```python
from build123d import *

# Parameters (mm, degrees)
FILLET4_R               = 3
CHAMFER1_SIZE2          = 0.393197641
CHAMFER1_SIZE           = 0.4
CUT_EXTRUDE1_DEPTH      = 10.487768718
CUT_EXTRUDE1_DEPTH_BACK = 12.0000001
FILLET5_R               = 0.4
FILLET6_R               = 2


with BuildPart() as part:
    # Sketch1 → Revolve1 (revolve)
    with BuildSketch(Plane.XY):
        Polygon((0, 1.95), (10.718918331, 1.95), (15.775669274, 0.5), (20.487768618, 0.58225), (20.487768618, 2.582554656), (16.03962094, 2.50491195), (11, 3.95), (11, 10), (8, 10), (8, 2.75), (0, 2.75), align=None)
    revolve(axis=Axis((0, 0, 0), (1, 0, 0)))

    # Fillet4
    fillet4_edges = [part.edges().sort_by_distance(p)[0] for p in [
        (15.775669274, -0.5, 0),
        (10.718918331, -1.95, 0),
    ]]
    fillet(fillet4_edges, radius=FILLET4_R)

    # Chamfer1
    chamfer1_edges = [part.edges().sort_by_distance(p)[0] for p in [
        (20.487768618, -2.582554656, 0),
    ]]
    chamfer(chamfer1_edges, length=CHAMFER1_SIZE, length2=CHAMFER1_SIZE2)

    # Sketch2 → Cut-Extrude1 (cut, two sides)
    with BuildSketch(Plane(origin=(11, 0, 0), x_dir=(0, 0, -1), z_dir=(1, 0, 0))) as cut_extrude1_sk:
        with BuildLine():
            Line((-10, 0), (-5, 8.660254038))
            ThreePointArc((-5, 8.660254038), (-8.660254038, 5), (-10, 0))
        make_face()
        with BuildLine():
            Line((-5, 8.660254038), (5, 8.660254038))
            ThreePointArc((5, 8.660254038), (0, 10), (-5, 8.660254038))
        make_face()
        with BuildLine():
            Line((5, 8.660254038), (10, 0))
            ThreePointArc((10, 0), (8.660254038, 5), (5, 8.660254038))
        make_face()
        with BuildLine():
            ThreePointArc((-10, 0), (-8.660254038, -5), (-5, -8.660254038))
            Line((-5, -8.660254038), (-10, 0))
        make_face()
        with BuildLine():
            ThreePointArc((-5, -8.660254038), (0, -10), (5, -8.660254038))
            Line((5, -8.660254038), (-5, -8.660254038))
        make_face()
        with BuildLine():
            ThreePointArc((5, -8.660254038), (8.660254038, -5), (10, 0))
            Line((10, 0), (5, -8.660254038))
        make_face()
    extrude(amount=CUT_EXTRUDE1_DEPTH, mode=Mode.SUBTRACT)
    extrude(cut_extrude1_sk.sketch, amount=-CUT_EXTRUDE1_DEPTH_BACK, mode=Mode.SUBTRACT)

    # Fillet5
    fillet5_edges = [part.edges().sort_by_distance(p)[0] for p in [
        (11, -4.330127019, -7.5),
        (8, -4.330127019, -7.5),
        (8, -8.660254038, 0),
        (8, 4.330127019, -7.5),
        (8, 4.330127019, 7.5),
        (9.5, 8.660254038, 5),
        (11, 4.330127019, 7.5),
        (9.5, 0, 10),
        (9.5, 0, -10),
        (11, 4.330127019, -7.5),
        (9.5, 8.660254038, -5),
        (9.5, -8.660254038, 5),
        (11, -8.660254038, 0),
        (9.5, -8.660254038, -5),
        (11, 8.660254038, 0),
        (8, 8.660254038, 0),
        (11, -4.330127019, 7.5),
        (8, -4.330127019, 7.5),
    ]]
    fillet(fillet5_edges, radius=FILLET5_R)

    # Fillet6
    fillet6_edges = [part.edges().sort_by_distance(p)[0] for p in [
        (11, -3.95, 0),
        (16.03962094, -2.50491195, 0),
    ]]
    fillet(fillet6_edges, radius=FILLET6_R)


solid = part.part
```
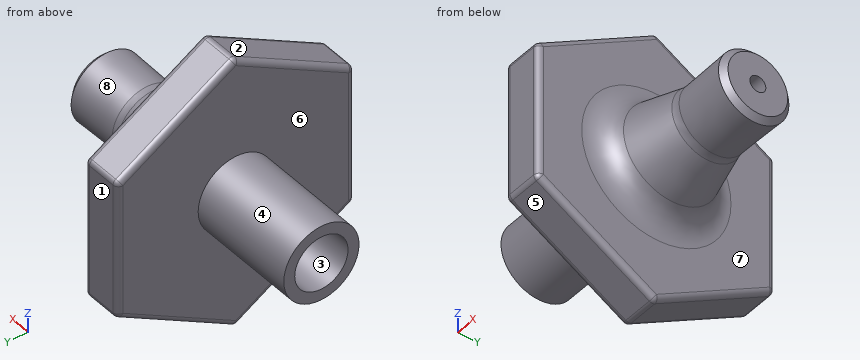
Model file for the job. Use its own axes, mm. Face numbers are marked on the shaded views. A direction names the side the tool comes from. Coordinates: 2 decimals unless noted, no trailing zeros. Write each loop counter-clockwise with the first axis right and the second up, starting at its lowest first coordinate (ties: lowest second). Pieces come first, ordered by that corner, then holes. Notation, with made-up numbers: (-16.5, 21) - (16.5, 21) arc R21 ccw to (16.5, 50) - close; hole circle Ø1 at (61.25, -4). An arc over 180 degrees is marked (long way). One line per question, with ' | ' between items. Start each with the question number.
Q1. Drill centre lines: line 1 (Z direction, x = 6, y = 0); line 2 (X direction, y = 2.25, z = -6.5); line 3 (Z direction, x = 10.25, y = 0.25). Where is each one in solid material? Low to high. Write a range as [from, to].
Q2. Pin check, flat tips, straight feed: pin 1 (3 mm diameter, centred on x = 17.5, z = 2.5, fed in from -Y); pin 2 (5 mm diameter, centred on y = 0, z = 0, fed in from +X); pin 3 (8 mm diameter, centred on y = 7, z = 5, fed in from -X); pin 4 (3 mm diameter, centred on x = 6, z = 7.5, fed in from -Y) (3 decimals). Stop position of each tip, or through.
Q3. Cut at B-B, the plane x = 3.5. List the corners of the cut face in (y, z), then the cut area to 3 significant figures.
Q4. Cut at C-C, the plane x = 19.25. List the corners of the cut face in (y, z).
Q5. Cut at A-A, the plane x = 9. List the corners of the cut face in (y, z), then the cut area to 3 significant figures.
Q6. Pull direction Y, two halves, no side cores. Call the marked faces 1, 2, 3 and 4: pulls with the +Y half, pulls with the -Y half, needs draft (parallel to the pull), parting line crosses it, or undercut.
Q7. 3-axis set-ups, long thin cutter, end or side, ignore diameter. For the marked faces 5, 6, 7 and 8: which of +Z, -Z, +X, -X, +Y, -Y reach the whole face in a straight line?
Answer below:
1) line 1: [-2.75, -1.95], [1.95, 2.75] | line 2: [8, 11] | line 3: [-9.86, -1.93], [1.93, 9.86]
2) pin 1: y = -2.33 | pin 2: x = 20.49 | pin 3: x = 8 | pin 4: through
3) outline: circle Ø5.5 at (0, 0); hole circle Ø3.9 at (0, 0) | area: 11.8 mm^2
4) outline: circle Ø5.12 at (0, 0); hole circle Ø1.12 at (0, 0)
5) outline: (-8.66, -4.77) arc R0.4 ccw to (-8.46, -5.12) - (-0.2, -9.88) arc R0.4 ccw to (0.2, -9.88) - (8.46, -5.12) arc R0.4 ccw to (8.66, -4.77) - (8.66, 4.77) arc R0.4 ccw to (8.46, 5.12) - (0.2, 9.88) arc R0.4 ccw to (-0.2, 9.88) - (-8.46, 5.12) arc R0.4 ccw to (-8.66, 4.77) - close; hole circle Ø3.9 at (0, 0) | area: 248 mm^2
6) face 1: pulls with the +Y half | face 2: pulls with the -Y half | face 3: undercut | face 4: parting line crosses it
7) face 5: -Z, +X, -X, -Y | face 6: -X | face 7: +X | face 8: none
